Source: three-view drawing plus pictorial views. Frame: mm from the lowest corner of the part. A direction names the side the tool comes from. Give positions to 0.01 mm unless a question says otherwise; leave off trailing zeros. Loops run counter-clockwise (first coordinate to the right, second up) from the corner with the lowest first, then second, coordinate; pieces in that order, holes last. Notation, with made-up numbers: M 1,36 L 29,36 A18 cw 29,69 Z; hole C 25.5,-2 d5. An arc over 180 degrees is marked long. Answer as a JSON object with one key per item and string values. Group by question number.
1) Access query for the marked faces 1 and 2. Directions: +Z, -Z, +X, -X, +Y, -Y. A direction counts if a zero-diameter tool reaches every point of the face in a straight line with its end or side. Return the directions, or none.
2) Section query A-A on x = 6.4. Return loops of the section in (y, z), plus the area to 3 significant figures.
3) Section query C-C on y = 24. Return loops of the section in (x, z).
4) Section query D-D on z = 13.25. Count the separate pieces of the cut face and the enclosed holes in it, plus the area to 3 significant figures.
5) First-contact query: P1, Ø6, axis at y = 14.5, z = 12.5, coming from the -X side; P2, Ø8, axis at x = 14, z = 19, coming from the +Y side; P3, Ø1, axis at y = 10, z = 18, coming from the +X side. Flat tips, straight axial feed; report the tip coordinate or a pass-through.
6) Section query B-B on z = 21.5. Return loops of the section in (x, y), plus the area to 3 significant figures.
7) Ray query, L1, parallel to Y at x = 24, z = 22.25; L2, parallel to Z at x = 5, y = 1. Return the intervals inside material, ascending.
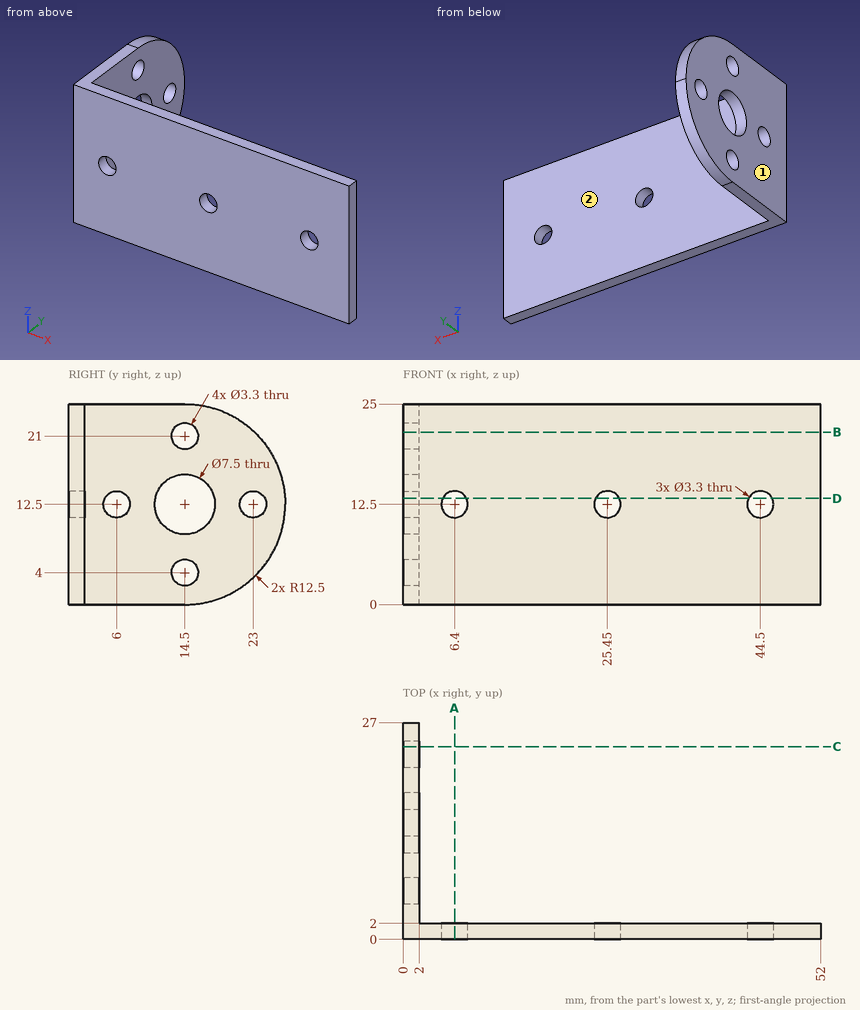
Output:
{
 "1": {"face 1": "+Z, -Z, -X, +Y, -Y", "face 2": "+Z, -Z, +X, +Y"},
 "2": {"outline": "M 0,0 L 2,0 L 2,10.85 L 0,10.85 Z; M 0,14.15 L 2,14.15 L 2,25 L 0,25 Z", "area": "43.4 mm^2"},
 "3": {"outline": "M 0,4.38 L 2,4.38 L 2,11.19 L 0,11.19 Z; M 0,13.81 L 2,13.81 L 2,20.62 L 0,20.62 Z"},
 "4": {"separate pieces": "7", "enclosed holes": "0", "area": "110 mm^2"},
 "5": {"P1": "passes through", "P2": "stops at y = 2", "P3": "stops at x = 2"},
 "6": {"outline": "M 0,0 L 52,0 L 52,2 L 2,2 L 2,12.93 L 0,12.93 Z; M 0,16.07 L 2,16.07 L 2,23.17 L 0,23.17 Z", "area": "140 mm^2"},
 "7": {"L1": "y = 0 to 2", "L2": "z = 0 to 11.63, 13.37 to 25"}
}
